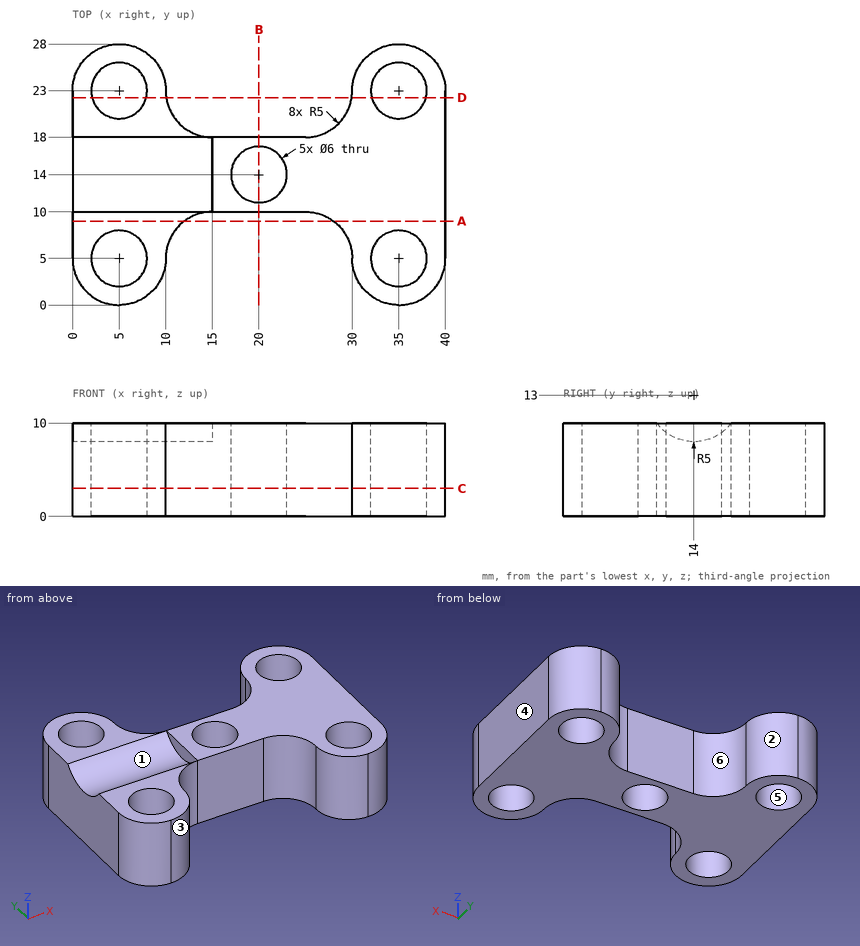
Part print with two shaded views. Sizes in mm from the minimum x, y, z corner. A direction names the side the tool comes from. Round coordinates to 2 decimals unless told otherwise and drop trailing zeros. Loops run counter-clockwise (first coordinate to the right, second up) from the corner with the lowest first, then second, coordinate; pieces in that order, holes last.
1. 3-axis set-ups, long thin cutter, end or side, ignore diameter. For the marked faces 1, 2 and 3: which of +Z, -Z, +X, -X, +Y, -Y reach the whole face in a straight line?
Solutions:
face 1: +Z, -X
face 2: +Z, -Z, +Y
face 3: +Z, -Z, -Y
2. Two-plate mould, pull along Y, no slides. Class the marked faces 4, 5 and 6: pulls with the +Y half, pulls with the -Y half, needs draft (parallel to the pull), parting line crosses it, or undercut.
Solutions:
face 4: needs draft
face 5: undercut
face 6: pulls with the +Y half
3. Drill centre lines: line 1 along X through (y, z) = (23, 6.75); line 2 along Y through (x, z) = (35, 4); line 3 along Y through (x, z) = (2.5, 6.75). Where is each one in solid material? Low to high.
Solutions:
line 1: x = 0 to 2, 8 to 10, 30 to 32, 38 to 40
line 2: y = 0 to 2, 8 to 20, 26 to 28
line 3: y = 0.67 to 3.34, 6.66 to 21.34, 24.66 to 27.33
4. Flat gauge pins, fed straight in: pin 1 (3 mm diameter, centred on x = 32.5, z = 9, fed in from +Y); pin 2 (3 mm diameter, centred on x = 18, z = 3, fed in from +Y); pin 3 (2 mm diameter, centred on y = 15, z = 9.5, fed in from -X). Where does each tip first touch, or does it go through?
Solutions:
pin 1: stops at y = 27.9
pin 2: stops at y = 18
pin 3: stops at x = 15
5. Slice it at C-C (z = 3). Count the separate pieces of the cut face and the enclosed holes in it, and give its area (3 significant figures).
Solutions:
separate pieces: 1
enclosed holes: 5
area: 557 mm2
6. Slice it at D-D (y = 22.25). Give the cut face in (x, z), and give its area (3 significant figures).
Solutions:
outline: (0, 0) - (2.1, 0) - (2.1, 10) - (0, 10) - close; (7.9, 0) - (10.06, 0) - (10.06, 10) - (7.9, 10) - close; (29.94, 0) - (32.1, 0) - (32.1, 10) - (29.94, 10) - close; (37.9, 0) - (40, 0) - (40, 10) - (37.9, 10) - close
area: 84.9 mm2
7. Slice it at B-B (x = 20). Give the cut face in (y, z), and give its area (3 significant figures).
Solutions:
outline: (10, 0) - (11, 0) - (11, 10) - (10, 10) - close; (17, 0) - (18, 0) - (18, 10) - (17, 10) - close
area: 20.0 mm2
8. Slice it at A-A (y = 9). Give the cut face in (x, z).
Solutions:
outline: (0, 0) - (12, 0) - (12, 10) - (0, 10) - close; (28, 0) - (40, 0) - (40, 10) - (28, 10) - close
